from build123d import *

# Parameters (mm, degrees)
SKETCH1_W                = 190
SKETCH1_H                = 100
BOSS_EXTRUDE1_DEPTH      = 3
BOSS_EXTRUDE2_DEPTH      = 95
BOSS_EXTRUDE2_DEPTH_BACK = 95
SKETCH2_W                = 3
SKETCH2_H                = 100
FILLET1_R                = 3
CUT_EXTRUDE1_DEPTH       = 30
CUT_EXTRUDE1_DEPTH_BACK  = 30
SKETCH3_R                = 2


with BuildPart() as part:
    # Sketch1 → Boss-Extrude1 (new body)
    with BuildSketch(Plane(origin=(0, 0, 0), x_dir=(1, 0, 0), z_dir=(0, 1, 0))):
        Rectangle(SKETCH1_W, SKETCH1_H)
    extrude(amount=BOSS_EXTRUDE1_DEPTH)

    # Sketch2 → Boss-Extrude2 (add, two sides: drawn at the far end of the back side and taken through both)
    with BuildSketch(Plane(origin=(0, 0, 0), x_dir=(0, 0, -1), z_dir=(1, 0, 0)).offset(-BOSS_EXTRUDE2_DEPTH_BACK)):
        with Locations((-48.5, 53)):
            Rectangle(SKETCH2_W, SKETCH2_H)
        Polygon((0, 23), (0, 27.8), (-47, 103), (-47, 98.2), align=None)
        Polygon((47, 98.2), (47, 103), (0, 27.8), (0, 23), align=None)
        with Locations((48.5, 53)):
            Rectangle(SKETCH2_W, SKETCH2_H)
    extrude(amount=BOSS_EXTRUDE2_DEPTH + BOSS_EXTRUDE2_DEPTH_BACK)

    # Fillet1
    # the kernel refuses this fillet: 3 mm, written as the material it adds along each edge
    with BuildSketch(Plane(origin=(-95, 27.8, 0), x_dir=(0, 0.8479983040050875, -0.529998940003181), z_dir=(1, 0, 0))) as fillet1_piece_1:
        with BuildLine():
            CenterArc((FILLET1_R * 1.6, FILLET1_R), FILLET1_R, 154.010766416, 115.989233584)
            Line((FILLET1_R * 0.701123595506, FILLET1_R * 1.43820224719), (0, 0))
            Line((0, 0), (FILLET1_R * 1.6, 0))
        make_face()
    extrude(amount=190)
    # the kernel refuses this fillet: 3 mm, written as the material it takes off along each edge
    with BuildSketch(Plane(origin=(-107, 23, 0), x_dir=(0, 0.8479983040050876, 0.5299989400031808), z_dir=(1, 0, 0))) as fillet1_2_piece_1:
        with BuildLine():
            CenterArc((FILLET1_R * 1.6, -FILLET1_R), FILLET1_R, 90, 115.989233584)
            Line((FILLET1_R * 0.701123595506, -FILLET1_R * 1.43820224719), (0, 0))
            Line((0, 0), (FILLET1_R * 1.6, 0))
        make_face()
    extrude(amount=214, mode=Mode.SUBTRACT)
    with BuildSketch(Plane(origin=(102.5, 103, 50), x_dir=(0, -1, 0), z_dir=(-1, 0, 0)), Plane(origin=(-102.5, 103, -50), x_dir=(0, -1, 0), z_dir=(1, 0, 0))) as fillet1_2_piece_2:
        with BuildLine():
            CenterArc((FILLET1_R, -FILLET1_R), FILLET1_R, 90, 90)
            Line((0, -FILLET1_R), (0, 0))
            Line((0, 0), (FILLET1_R, 0))
        make_face()
    extrude(amount=205, mode=Mode.SUBTRACT)
    with BuildSketch(Plane(origin=(99.156857311, 103, 47), x_dir=(0, 0, 1), z_dir=(-1, 0, 0)), Plane(origin=(-99.156857311, 103, -47), x_dir=(0, 0, -1), z_dir=(1, 0, 0))) as fillet1_2_piece_3:
        with BuildLine():
            CenterArc((FILLET1_R * 0.554247641507, -FILLET1_R), FILLET1_R, 90, 57.994616792)
            Line((-FILLET1_R * 0.293750662498, -FILLET1_R * 0.470001059997), (0, 0))
            Line((0, 0), (FILLET1_R * 0.554247641507, 0))
        make_face()
    extrude(amount=198.313714623, mode=Mode.SUBTRACT)

    # Sketch3 → Cut-Extrude1 (cut, two sides: drawn at the far end of the back side and taken through both)
    with BuildSketch(Plane.XY.offset(-CUT_EXTRUDE1_DEPTH_BACK)):
        with Locations(Location((0, 50, 0), (0, 0, 270))):
            Circle(SKETCH3_R)
    extrude(amount=CUT_EXTRUDE1_DEPTH + CUT_EXTRUDE1_DEPTH_BACK, mode=Mode.SUBTRACT)


solid = part.part
Input: part model. Units: mm. Frame: model coordinates. A direction names the side the tool comes from. Coordinates: 2 decimals unless noted, no trailing zeros. Order: outer loops, then holes, each group sorted by start corner. A loop starts at its lowest first (then second) coordinate and runs counter-clockwise, first axis right, second up. Notation, with made-up numbers: M -25.75,88.5 L 25.25,88.5 A6 ccw 25.25,93.5 Z; hole C 78.25,60.5 d9. An arc over 180 degrees is marked long. Write item = value, one per line. Start each with the question number.
(1) Reachability of faces 4 (the flat face through (-1.33, 67.218, -24.636)), 5 (the cylindrical face through (-0.766, 48.153, 15.394)), 6 (the flat face through (-1, 50, -47)), 7 (the flat face through (-1, 49, -50)) from +Z, -Z, +X, -X, +Y, -Y: full face, straight path, thin tool, end or side. Return the list, or none.
(2) Line query: line 1 along Z through (x, y) = (-32, 15); line 2 along Z through (x, y) = (-41, 52.5); line 3 along Z through (x, y) = (-37, 44.5). Output: solid intervals per line, ascending. Write a range as [from, to].
(3) Section D-D on y = 86. Output: boundary loops of the cut face in (x, z) (3 decimals), and give its area (3 significant figures).
(4) Section B-B on z = -21.5. Output: boundary loops of the cut face in (x, y).
(5) Section A-A on y = 8.5. Output: boundary loops of the cut face in (x, z).
(6) First-contact query: P1, Ø3, axis at x = 20, z = 34, coming from the +Y side; P2, Ø12, axis at x = 61, z = -12, coming from the +Y side; P3, Ø12, axis at x = -17, z = 3.5, coming from the +Y side. Flat tips, straight axial feed; report the tip coordinate or a pass-through.
(7) Pull-direction query (X, two-part tool) for faces 1 (the flat face through (95, 38, 8)), 2 (the flat face through (-1.3, 66.2, 24)), 3 (the cylindrical face through (0.601, 48.092, -15.473)); classes: released by +X, released by -X, zero draft, split by the parting line, or undercut.
(8) Section C-C on x = 33. Output: boundary loops of the cut face in (y, z).
Result set:
q1.face_4 = +X, -X, +Y
q1.face_5 = none
q1.face_6 = +X, -X
q1.face_7 = -Z, +X, -X, +Y, -Y
q2.line_1 = [-50, -47], [47, 50]
q2.line_2 = [-50, -47], [-18.44, -15.44], [15.44, 18.44], [47, 50]
q2.line_3 = [-50, -47], [-13.44, -10.44], [10.44, 13.44], [47, 50]
q3.outline = M -95,-50 L 95,-50 L 95,-47 L -95,-47 Z; M -95,-39.375 L 95,-39.375 L 95,-36.375 L -95,-36.375 Z; M -95,36.375 L 95,36.375 L 95,39.375 L -95,39.375 Z; M -95,47 L 95,47 L 95,50 L -95,50 Z
q3.area = 2,280 mm²
q4.outline = M -95,0 L 95,0 L 95,3 L -95,3 Z; M -95,57.4 L 95,57.4 L 95,62.2 L -95,62.2 Z
q5.outline = M -95,-50 L 95,-50 L 95,-47 L -95,-47 Z; M -95,47 L 95,47 L 95,50 L -95,50 Z
q6.P1 = 84.6
q6.P2 = 56.6
q6.P3 = 43
q7.face_1 = released by +X
q7.face_2 = zero draft
q7.face_3 = undercut
q8.outline = M 0,-50 L 100,-50 A3 ccw 102.88,-47.83 A3 ccw 101.59,-46.12 L 31.87,-2.54 A3 cw 31.87,2.54 L 101.59,46.12 A3 ccw 102.88,47.83 A3 ccw 100,50 L 0,50 Z; hole M 3,-47 L 98.2,-47 L 27.07,-2.54 A3 cw 27.07,2.54 L 98.2,47 L 3,47 Z
